Geometry: final body of the model. Coordinates: model frame, mm. A direction names the side the tool comes from. Give positions to 0.01 mm unless a question says otherwise; leave off trailing zeros. Order: outer loops, then holes, each group sorted by start corner. A loop starts at its lowest first (then second) coordinate and runs counter-clockwise, first axis right, second up. Notation, with made-up numbers: (27, -28.5) -> (63, -28.5) arc R27 cw to (63, 7.5) -> close; hole circle Ø6 at (-12, 36). An arc over 180 degrees is marked (long way). Write item = value, one per line.
```python
from build123d import *

# Parameters (mm, degrees)
SKETCH1_W          = 60.3
SKETCH1_H          = 50.1
OUTERWALLS_DEPTH   = 2
SKETCH2_W          = 60.3
SKETCH2_H          = 50.1
SKETCH2_W_2        = 57.9
SKETCH2_H_2        = 47.7
INNER_DEPTH        = 2.1
SKETCH4_W          = 10
SKETCH4_H          = 3.7
CUT_EXTRUDE1_DEPTH = 20
FILLET1_R          = 2


with BuildPart() as part:
    # Sketch1 → OuterWalls (new body)
    with BuildSketch(Plane(origin=(0, 0, 0), x_dir=(1, 0, 0), z_dir=(0, 1, 0))):
        Rectangle(SKETCH1_W, SKETCH1_H)
    extrude(amount=-OUTERWALLS_DEPTH)

    # Sketch2 → Inner (add)
    with BuildSketch(Plane(origin=(0, -2, 0), x_dir=(-1, 0, 0), z_dir=(0, -1, 0))):
        Rectangle(SKETCH2_W, SKETCH2_H)
        Rectangle(SKETCH2_W_2, SKETCH2_H_2, mode=Mode.SUBTRACT)
    extrude(amount=INNER_DEPTH)

    # Sketch4 → Cut-Extrude1 (cut)
    with BuildSketch(Plane(origin=(30.15, 0, 0), x_dir=(0, 0, -1), z_dir=(1, 0, 0))):
        with Locations((4.91675286, -5.05)):
            Rectangle(SKETCH4_W, SKETCH4_H)
    extrude(amount=-CUT_EXTRUDE1_DEPTH, mode=Mode.SUBTRACT)

    # Fillet1
    fillet1_edges = [part.edges().sort_by_distance(p)[0] for p in [
        (0, 0, -25.05),
        (30.15, 0, 0),
        (0, 0, 25.05),
        (-30.15, 0, 0),
        (-30.15, -2.05, -25.05),
        (30.15, -2.05, -25.05),
        (30.15, -2.05, 25.05),
        (-30.15, -2.05, 25.05),
    ]]
    fillet(fillet1_edges, radius=FILLET1_R)


solid = part.part
```
1) First-contact query: P1, Ø1, axis at x = 30, y = -3.5, coming from the +Z side; P2, Ø1, axis at x = 29.5, z = -5.5, coming from the -Y side. Flat tips, straight axial feed; report the tip coordinate or a pass-through.
Check sheet entries:
P1 = 24.53
P2 = -3.2
2) Section query B-B (x = 22.5). Output: boundary loops of the cut face in (y, z), plus the area to 3 significant figures.
Check sheet entries:
outline = (-4.1, -25.05) -> (-2, -25.05) arc R2 ccw to (0, -23.05) -> (0, 23.05) arc R2 ccw to (-2, 25.05) -> (-4.1, 25.05) -> (-4.1, 23.85) -> (-2, 23.85) -> (-2, -23.85) -> (-4.1, -23.85) -> close
area = 104 mm²
3) Section query A-A (z = 4). Output: boundary loops of the cut face in (x, y).
Check sheet entries:
outline = (-30.15, -4.1) -> (-28.95, -4.1) -> (-28.95, -2) -> (28.95, -2) -> (28.95, -4.1) -> (30.15, -4.1) -> (30.15, -2) arc R2 ccw to (28.15, 0) -> (-28.15, 0) arc R2 ccw to (-30.15, -2) -> close
4) Reachability of faces 1 (the face through (29.6, -3.2, -4.8)), 2 (the face through (-29.55, -0.57, -0.32)), 3 (the face through (-28.95, -3, 0)) from +Z, -Z, +X, -X, +Y, -Y: full face, straight path, thin tool, end or side. Return the list, or none.
Check sheet entries:
face_1 = +X, -Y
face_2 = +Z, -Z, -X, +Y
face_3 = -Y
5) Line query: line 1 (X direction, y = -3.3, z = -15.5); line 2 (Z direction, x = -5.5, y = -2.6); line 3 (Y direction, x = 9, z = -16). Output: solid intervals per line, ascending. Write a range as from..to.
Check sheet entries:
line_1 = -30.15..-28.95, 28.95..30.15
line_2 = -25.05..-23.85, 23.85..25.05
line_3 = -2..0
